from build123d import *

# Parameters (mm, degrees)
F0_R     = 2.6
F1_DEPTH = 3
F2_R     = 5
F3_R     = 2.6
F3_W     = 8
F3_H     = 15
F4_DEPTH = 2
F5_SIZE  = 1


with BuildPart() as f1:
    # F0 (on Top) → F1 (new body)
    with BuildSketch(Plane.XY):
        with BuildLine():
            Line((30, 0), (0, 0))
            Line((0, 0), (0, 30))
            Line((0, 30), (-9.065466, 30))
            ThreePointArc((-9.065466, 30), (-16.222051, 11.49184), (-30.6, -2.184537))
            Line((-30.6, -2.184537), (-30.6, -15))
            Line((-30.6, -15), (30, -15))
            Line((30, -15), (30, 0))
        make_face()
        with Locations((-21.4, -7.643007)):
            Circle(F0_R, mode=Mode.SUBTRACT)
        with Locations((8.5, -7.643007)):
            Circle(F0_R, mode=Mode.SUBTRACT)
    extrude(amount=F1_DEPTH)

    # F2
    f2_edges = [f1.edges().sort_by_distance(p)[0] for p in [
        (-30.6, -15, 1.5),
        (-30.6, -2.184537, 1.5),
        (30, -15, 1.5),
        (-9.065466, 30, 1.5),
    ]]
    fillet(f2_edges, radius=F2_R)

    # F3 (on face) → F4 (join)
    with BuildSketch(Plane.XY):
        with BuildLine():
            Line((-25.4, 1.447635), (-25.4, -15))
            Line((-25.4, -15), (-17.4, -15))
            Line((-17.4, -15), (-17.4, 9.814667))
            ThreePointArc((-17.4, 9.814667), (-21.131748, 5.374666), (-25.4, 1.447635))
        make_face()
        with Locations((-21.4, -7.643007)):
            Circle(F3_R, mode=Mode.SUBTRACT)
        with Locations((8.5, -7.5)):
            Rectangle(F3_W, F3_H)
        with Locations((8.5, -7.643007)):
            Circle(F3_R, mode=Mode.SUBTRACT)
    extrude(amount=-F4_DEPTH)

    # F5
    f5_edges = [f1.edges().sort_by_distance(p)[0] for p in [
        (-25.4, -6.776183, -2),
        (-17.4, -2.592667, -2),
        (4.5, -7.5, -2),
        (12.5, -7.5, -2),
    ]]
    chamfer(f5_edges, length=F5_SIZE)


solid = f1.part
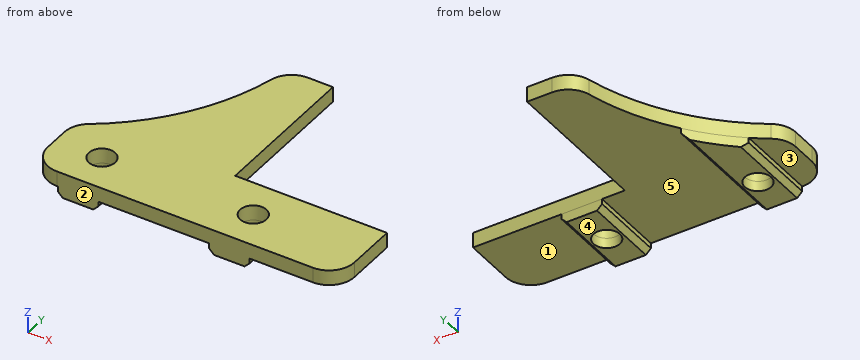
The model under review builds one solid part; all positions refer to its coordinate system, in mm. Face numbers are marked on the shaded views. A direction names the side the tool comes from. Give positions to 0.01 mm unless a question says otherwise; leave off trailing zeros. Loops run counter-clockwise (first coordinate to the right, second up) from the corner with the lowest first, then second, coordinate; pieces in that order, holes last. Notation, with made-up numbers: (6, -24) -> (65, -24) arc R15 cw to (65, -1) -> close; hole circle Ø6 at (79.5, -32.75). An arc over 180 degrees is marked (long way). Write each question's results on one line, items separated by ' | '.
1) Take a section at A-A, the plane x = 8.5. Give the boundary of the cut face in (y, z), plus the area to 3 significant figures.
Conclusion:
outline: (-15, -2) -> (-10.24, -2) -> (-10.24, 3) -> (-15, 3) -> close; (-5.04, -2) -> (0, -2) -> (0, 3) -> (-5.04, 3) -> close | area: 49.0 mm^2
2) For line 1 along Y through (x, z) = (8.5, -1.2); line 2 along X through (y, z) = (-6, 0.4); line 3 along Z through (x, y) = (-5, 15), list the stretches that pass through material, from the lowest coordinate up. Write a range as from..to.
Conclusion:
line 1: y = -15..-10.24, -5.04..0 | line 2: x = -30.6..-23.42, -19.38..6.48, 10.52..30 | line 3: z = 0..3
3) Take a section at C-C, the plane y = -3.5. Give the boundary of the cut face in (x, z), plus the area to 3 significant figures.
Conclusion:
outline: (-30.39, 0) -> (-25.4, 0) -> (-25.4, -1) -> (-24.4, -2) -> (-18.4, -2) -> (-17.4, -1) -> (-17.4, 0) -> (4.5, 0) -> (4.5, -1) -> (5.5, -2) -> (11.5, -2) -> (12.5, -1) -> (12.5, 0) -> (30, 0) -> (30, 3) -> (-30.39, 3) -> close | area: 211 mm^2
4) Take a section at B-B, the plane z = 2.15. Give the boundary of the cut face in (x, y).
Conclusion:
outline: (-30.6, -10) arc R5 ccw to (-25.6, -15) -> (25, -15) arc R5 ccw to (30, -10) -> (30, 0) -> (0, 0) -> (0, 30) -> (-4.95, 30) arc R5 ccw to (-9.81, 26.16) arc R45.32 cw to (-28.41, -0.79) arc R5 ccw to (-30.6, -4.92) -> close; hole circle Ø5.2 at (-21.4, -7.64); hole circle Ø5.2 at (8.5, -7.64)
5) Draft analysis for pull direction X (two halves, no side actions). For the marked faces 4 and 5, state which applies: pulls with the +X half, pulls with the -X half, needs draft (parallel to the pull), parting line crosses it, or undercut.
Conclusion:
face 4: needs draft | face 5: undercut
6) Tool access review of the marked faces 1, 2 and 3: name each direction out of +Z, -Z, +X, -X, +Y, -Y from which nothing blocks a thin tool from reaching the whole face with its end or side.
Conclusion:
face 1: -Z, +X, +Y, -Y | face 2: +Z, -Z, +X, -X, -Y | face 3: -Z, -X, +Y, -Y
7) Take a section at D-D, the plane x = -21.4. Give the boundary of the cut face in (y, z), plus the area to 3 significant figures.
Conclusion:
outline: (-15, -2) -> (-10.24, -2) -> (-10.24, 3) -> (-15, 3) -> close; (-5.04, -2) -> (5.1, -2) -> (5.1, 3) -> (-5.04, 3) -> close | area: 74.5 mm^2
8) Insertion check: pin 1 Ø1.6 at (x, z) = (10.5, -1) entering from +Y; pin 2 Ø12 at (x, y) = (-8, 5) entering from -Z; pin 3 Ø0.8 at (y, z) = (-9.5, -0.5) entering from -X. Each pin has a flat end and moves straight along its axis. Give the tip position at first contact, or say it passes through.
Conclusion:
pin 1: stops at y = 0 | pin 2: stops at z = 0 | pin 3: stops at x = -25.4
